Drawing for the job (mm, zero at the part's lowest x, y, z). A direction names the side the tool comes from. Round coordinates to 2 decimals unless told otherwise and drop trailing zeros. Loops run counter-clockwise (first coordinate to the right, second up) from the corner with the lowest first, then second, coordinate; pieces in that order, holes last. Notation, with made-up numbers: (16, 7.25) - (37, 7.25) arc R24 cw to (37, 46.25) - close; hole circle Ø5 at (87, 30). An arc over 180 degrees is marked (long way). Put each result on its own line as item: value.
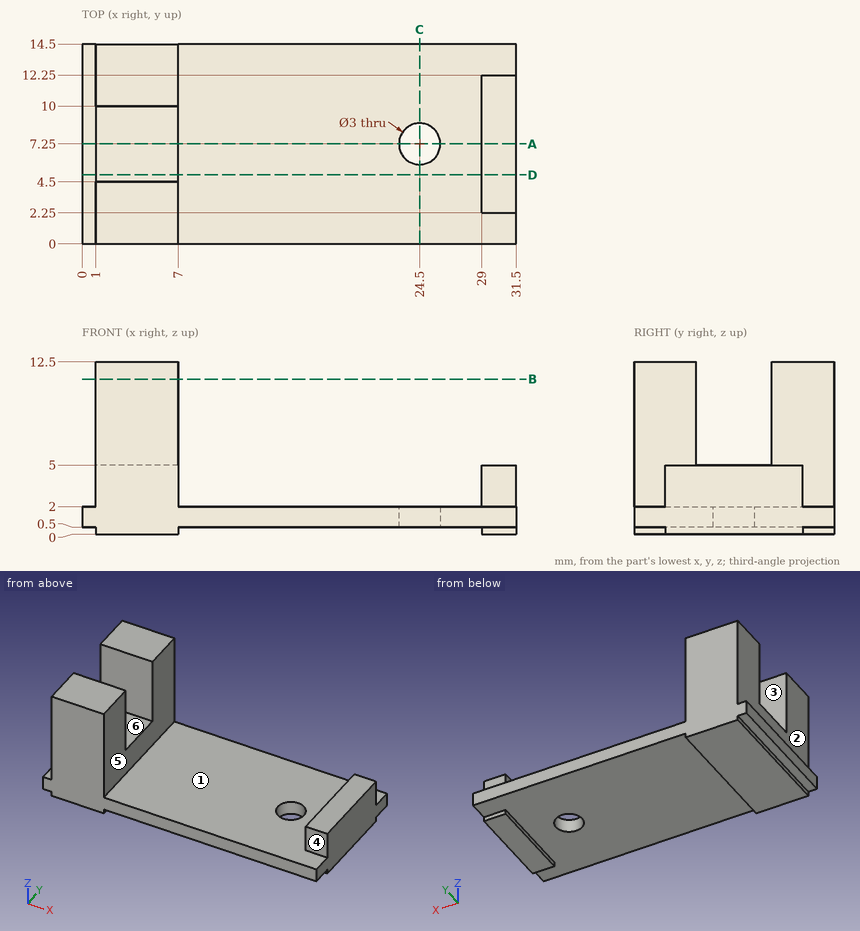
1. Two-plate mould, pull along X, no slides. Class the marked faces 1, 2 and 3: pulls with the +X half, pulls with the -X half, needs draft (parallel to the pull), parting line crosses it, or undercut.
A:
face 1: undercut
face 2: pulls with the -X half
face 3: needs draft
2. Band-saw the part on B-B (z = 11.25). List the corners of the cut face in (x, y).
A:
outline: (1, 0) - (7, 0) - (7, 4.5) - (1, 4.5) - close; (1, 10) - (7, 10) - (7, 14.5) - (1, 14.5) - close
3. Tool access for the marked faces 4, 5 and 6: list every direction of +Z, -Z, +X, -X, +Y, -Y with a clear straight run to the whole face (end or side of a thin tool).
A:
face 4: +Z, +X, -Y
face 5: +Z, +Y, -Y
face 6: +Z, +X, -X
4. Probe line 1 along Y through (x, z) = (24.5, 1.1); line 2 along X through (y, z) = (7, 3.25); line 3 along Z through (x, y) = (18.5, 1). List the from-to ranges inside material, lowest first. Write a range as [from, to].
A:
line 1: y = [0, 5.75], [8.75, 14.5]
line 2: x = [1, 7], [29, 31.5]
line 3: z = [0.5, 2]
5. Band-saw the part on A-A (y = 7.25). List the corners of the cut face in (x, z).
A:
outline: (0, 0.5) - (1, 0.5) - (1, 0) - (7, 0) - (7, 0.5) - (23, 0.5) - (23, 2) - (7, 2) - (7, 5) - (1, 5) - (1, 2) - (0, 2) - close; (26, 0.5) - (29, 0.5) - (29, 0) - (31.5, 0) - (31.5, 5) - (29, 5) - (29, 2) - (26, 2) - close
6. Band-saw the part on D-D (y = 5). List the corners of the cut face in (x, z), plus the area to 3 significant figures.
A:
outline: (0, 0.5) - (1, 0.5) - (1, 0) - (7, 0) - (7, 0.5) - (29, 0.5) - (29, 0) - (31.5, 0) - (31.5, 5) - (29, 5) - (29, 2) - (7, 2) - (7, 5) - (1, 5) - (1, 2) - (0, 2) - close
area: 77.0 mm²
7. Band-saw the part on C-C (x = 24.5). List the corners of the cut face in (y, z).
A:
outline: (0, 0.5) - (5.75, 0.5) - (5.75, 2) - (0, 2) - close; (8.75, 0.5) - (14.5, 0.5) - (14.5, 2) - (8.75, 2) - close
8. Pin check, flat tips, straight feed: P1, Ø0.8, axis at x = 0.5, y = 9.5, coming from the -Z side; P2, Ø3, axis at y = 9, z = 10, coming from the +X side; P3, Ø3, axis at x = 30.5, y = 9, coming from the +Z side. Stop position of each tip, or through.
A:
P1: stops at z = 0.5
P2: stops at x = 7
P3: stops at z = 5
